Here's how the part is built. I have some questions about the finished solid (model axes, mm). A direction names the side the tool comes from. Give positions to 0.01 mm unless a question says otherwise; leave off trailing zeros. Loops run counter-clockwise (first coordinate to the right, second up) from the corner with the lowest first, then second, coordinate; pieces in that order, holes last. Notation, with made-up numbers: (81, -18) - (128, -18) arc R25 cw to (128, 8) - close; hole circle Ø6 at (-27.5, -25.75). An arc over 180 degrees is marked (long way). Use a Markdown table: item, result.
from build123d import *

# Parameters (mm, degrees)
EXTRUDE_1_DEPTH = 4.5
EXTRUDE_2_DEPTH = 0.3


with BuildPart() as part:
    # Эскиз1 → Бобышка-Вытянуть1 (new body)
    with BuildSketch(Plane(origin=(0, 0, 0), x_dir=(1, 0, 0), z_dir=(0, 1, 0))):
        with BuildLine():
            Line((-2.024845673, -1.55), (2.024845673, -1.55))
            ThreePointArc((2.024845673, -1.55), (0, 2.55), (-2.024845673, -1.55))
        make_face()
    extrude(amount=EXTRUDE_1_DEPTH)

    # Эскиз3 → Бобышка-Вытянуть2 (add, symmetric)
    with BuildSketch(Plane.XY):
        Polygon((-0.375, 0), (0.375, 0), (0.375, -1.2), (0.5, -1.2), (0.5, -2.2), (0.375, -2.2), (0.375, -5.2), (-0.375, -5.2), (-0.375, -2.2), (-0.5, -2.2), (-0.5, -1.2), (-0.375, -1.2), align=None)
        Polygon((0.895, 0), (1.645, 0), (1.645, -1.2), (1.77, -1.2), (1.77, -2.2), (1.645, -2.2), (1.645, -5.2), (0.895, -5.2), (0.895, -2.2), (0.77, -2.2), (0.77, -1.2), (0.895, -1.2), align=None)
        Polygon((-1.77, -1.2), (-1.77, -2.2), (-1.645, -2.2), (-1.645, -5.2), (-0.895, -5.2), (-0.895, -2.2), (-0.77, -2.2), (-0.77, -1.2), (-0.895, -1.2), (-0.895, 0), (-1.645, 0), (-1.645, -1.2), align=None)
    extrude(amount=EXTRUDE_2_DEPTH, both=True)


solid = part.part
(1) Suppose I cut it at A-A on y = -2. Write out the boundary of the cut face in (x, z).
A:
| item | result |
|---|---|
| outline | (-1.77, -0.3) - (-0.77, -0.3) - (-0.77, 0.3) - (-1.77, 0.3) - close; (-0.5, -0.3) - (0.5, -0.3) - (0.5, 0.3) - (-0.5, 0.3) - close; (0.77, -0.3) - (1.77, -0.3) - (1.77, 0.3) - (0.77, 0.3) - close |
(2) On a 3-axis mill with a long thin cutter (end or side, diameter ignored), from which of +Z, -Z, +X, -X, +Y, -Y can I reach the whole of each face in a straight line? I mean faces 1 (the face through (0, 2, 1.55)), 2 (the face through (-1.3, -2.6, -0.3)), 3 (the face through (-1.3, -2.6, 0.3)). Say none if no direction works.
A:
| item | result |
|---|---|
| face 1 | +Z, +X, -X, +Y, -Y |
| face 2 | -Z, +X, -X, -Y |
| face 3 | +Z, +X, -X, -Y |
(3) Suppose I cut it at B-B on x = -1.3. Write out the boundary of the cut face in (y, z).
A:
| item | result |
|---|---|
| outline | (-5.2, -0.3) - (0, -0.3) - (0, -2.19) - (4.5, -2.19) - (4.5, 1.55) - (0, 1.55) - (0, 0.3) - (-5.2, 0.3) - close |
(4) Will these pins go through, and if not, where does the flat tip stop? pin 1 (0.5 mm diameter, centred on y = -4, z = 0, fed in from -X) (3 decimals); pin 2 (0.7 mm diameter, centred on y = -2, z = 0, fed in from -X); pin 3 (1.5 mm diameter, centred on x = 1, y = -4, fed in from +Z); pin 4 (2 mm diameter, centred on x = 1, y = 1, fed in from -Z).
A:
| item | result |
|---|---|
| pin 1 | x = -1.645 |
| pin 2 | x = -1.77 |
| pin 3 | z = 0.3 |
| pin 4 | z = -2.55 |
(5) Suppose I cut it at C-C on y = -3.25. Write out the boundary of the cut face in (x, z) (3 decimals), plus the area to 3 significant figures.
A:
| item | result |
|---|---|
| outline | (-1.645, -0.3) - (-0.895, -0.3) - (-0.895, 0.3) - (-1.645, 0.3) - close; (-0.375, -0.3) - (0.375, -0.3) - (0.375, 0.3) - (-0.375, 0.3) - close; (0.895, -0.3) - (1.645, -0.3) - (1.645, 0.3) - (0.895, 0.3) - close |
| area | 1.35 mm2 |
(6) Suppose I cut it at D-D on z = -1.6. Write out the boundary of the cut face in (x, y).
A:
| item | result |
|---|---|
| outline | (-1.99, 0) - (1.99, 0) - (1.99, 4.5) - (-1.99, 4.5) - close |
(7) If I drill on line 1 (Y direction, x = -1, z = 0.85); line 2 (Z direction, x = 0.95, y = -2.75); line 3 (X direction, y = 0.25, z = -1.5), over which ranges is the centre line in solid material (lowest first)?
A:
| item | result |
|---|---|
| line 1 | 0 to 4.5 |
| line 2 | -0.3 to 0.3 |
| line 3 | -2.06 to 2.06 |
